For this review, use the dimensioned drawing (mm, ordinates from the lowest corner) and the shaded views. Coordinates: 2 decimals unless noted, no trailing zeros. Loops run counter-clockwise (first coordinate to the right, second up) from the corner with the lowest first, then second, coordinate; pieces in that order, holes last. Notation, with made-up numbers: (-21.5, -40) - (-9.5, -40) arc R20 cw to (-9.5, -1) - close; hole circle Ø9 at (69.25, 88). An arc over 180 degrees is marked (long way). One line per item, written item: value. Start each with the question number.
1. Insertion check: P1, Ø8.5, axis at x = 150.78, y = 6.35, coming from the -Z side (3 decimals). The pin has a flat end and moves straight along its axis. Give the tip position at first contact, or say it passes through.
2. To check wall thickness, follow line 1 (X direction, y = 13.5, z = 25.5) (1 decimal); line 2 (Z direction, x = 142, y = 6.75) (1 decimal); line 3 (Y direction, x = 236, z = 32.5) (1 decimal). State the ranges of each line that lie inside material, in increasing order.
3. We need section C-C, the plane x = 81. Give the boundary of the cut face in (y, z) (1 decimal), then the cut area to 3 significant figures.
4. Mouldability with a two-part tool opening along Y and no side actions: class the marked faces 1 and 2 as +Y half, -Y half, draft (parallel to the pull), parting line (faces both ways), or undercut.
5. We need section D-D, the plane z = 72. Give the boundary of the cut face in (x, y) (1 decimal).
6. We need section A-A, the plane z = 57.15. Give the boundary of the cut face in (x, y) (1 decimal), then the cut area to 3 significant figures.
7. We need section B-B, the plane y = 6.35. Count the separate pieces of the cut face and the enclosed holes in it, then the cut area to 3 significant figures.
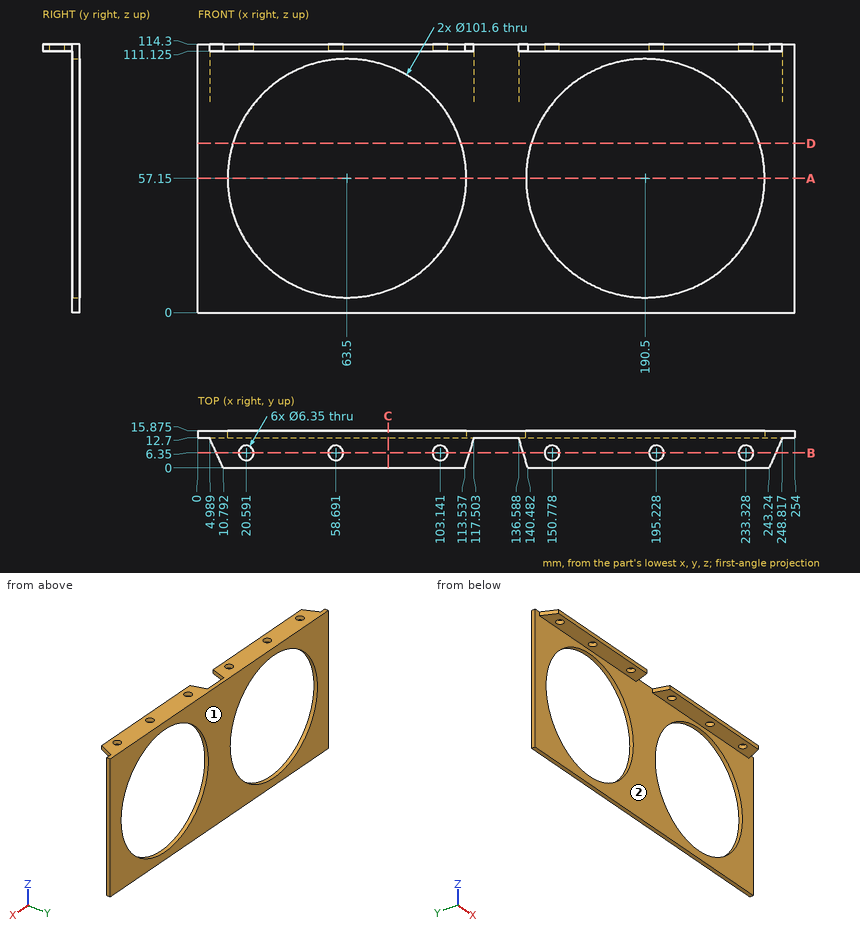
Findings below:
1. P1: z = 111.125
2. line 1: 0 to 23.8, 103.2 to 150.8, 230.2 to 254
2. line 2: 111.1 to 114.3
2. line 3: 12.7 to 15.9
3. outline: (0, 111.1) - (12.7, 111.1) - (12.7, 104.8) - (15.9, 104.8) - (15.9, 114.3) - (0, 114.3) - close; (12.7, 0) - (15.9, 0) - (15.9, 9.5) - (12.7, 9.5) - close
3. area: 100 mm2
4. face 1: +Y half
4. face 2: -Y half
5. outline: (0, 12.7) - (14.9, 12.7) - (14.9, 15.9) - (0, 15.9) - close; (112.1, 12.7) - (141.9, 12.7) - (141.9, 15.9) - (112.1, 15.9) - close; (239.1, 12.7) - (254, 12.7) - (254, 15.9) - (239.1, 15.9) - close
6. outline: (0, 12.7) - (12.7, 12.7) - (12.7, 15.9) - (0, 15.9) - close; (114.3, 12.7) - (139.7, 12.7) - (139.7, 15.9) - (114.3, 15.9) - close; (241.3, 12.7) - (254, 12.7) - (254, 15.9) - (241.3, 15.9) - close
6. area: 161 mm2
7. separate pieces: 8
7. enclosed holes: 0
7. area: 562 mm2
